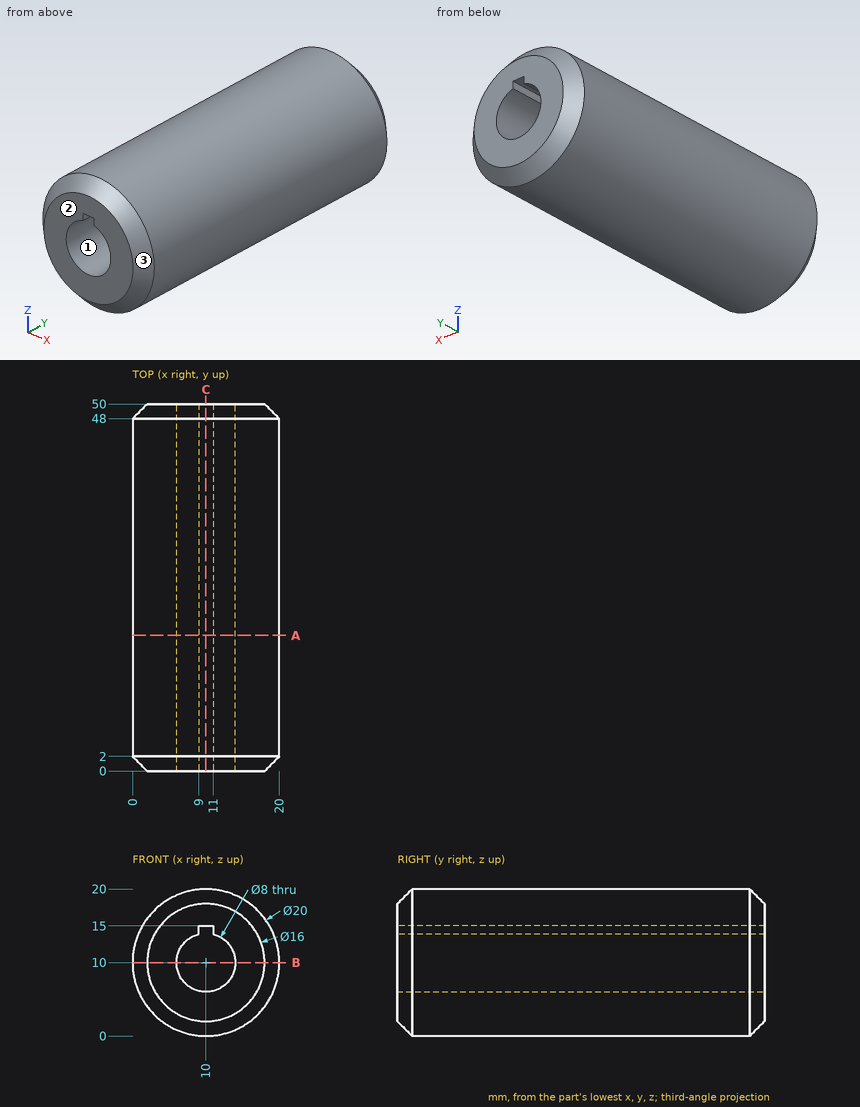
For this review, use the dimensioned drawing (mm, ordinates from the lowest corner) and the shaded views. Give positions to 0.01 mm unless a question says otherwise; leave off trailing zeros. Write each loop counter-clockwise with the first axis right and the second up, starting at its lowest first coordinate (ties: lowest second). Pieces come first, ordered by that corner, then holes.
(1) To check wall thickness, follow L1, parallel to Z at x = 10, y = 39.5; L2, parallel to Z at x = 8.5, y = 9; L3, parallel to X at y = 42, z = 18.75. State the ranges of each line that lie inside material, in increasing order.
(2) Consider section B-B, the plane z = 10. Give the boundary of the cut face in (x, y).
(3) Consider section A-A, the plane y = 18.5. Give the boundary of the cut face in (x, z).
(4) For P1, Ø6, axis at y = 34.5, z = 3.5, coming from the -X side; P2, Ø1.5, axis at y = 21.5, z = 3, coming from the -X side; P3, Ø3, axis at x = 15.5, y = 29, coming from the -Z side; P4, Ø3, axis at x = 15.5, z = 11.5, coming from the -Y side, all flat-tipped, find the tip position at first contact; note any pin that passes through.
(5) The part is to be moulded in two halves that separate along X. For the marked faces 1, 2 and 3, say which applies: released by +X, released by -X, zero draft, split by the parting line, or undercut.
(6) Consider section C-C, the plane x = 10. Give the boundary of the cut face in (y, z).
Returned:
1. L1: z = 0 to 6, 15 to 20
1. L2: z = 0.11 to 6.29, 13.71 to 19.89
1. L3: x = 5.16 to 14.84
2. outline: (0, 2) - (2, 0) - (6, 0) - (6, 50) - (2, 50) - (0, 48) - close; (14, 0) - (18, 0) - (20, 2) - (20, 48) - (18, 50) - (14, 50) - close
3. outline: circle Ø20 at (10, 10); hole (9, 13.87) arc R4 ccw (long way) to (11, 13.87) - (11, 15) - (9, 15) - close
4. P1: stops at x = 0.63
4. P2: stops at x = 2.19
4. P3: stops at z = 0.83
4. P4: stops at y = 0
5. face 1: undercut
5. face 2: zero draft
5. face 3: split by the parting line
6. outline: (0, 2) - (2, 0) - (48, 0) - (50, 2) - (50, 6) - (0, 6) - close; (0, 15) - (50, 15) - (50, 18) - (48, 20) - (2, 20) - (0, 18) - close
